For this review, take the finished solid that the model builds, in its own axes (mm). Coordinates: 2 decimals unless noted, no trailing zeros. Loops run counter-clockwise (first coordinate to the right, second up) from the corner with the lowest first, then second, coordinate; pieces in that order, holes last. Notation, with made-up numbers: (11.5, -37) -> (16.5, -37) arc R27 ccw to (16.5, -16) -> close; hole circle Ø4 at (17, 4.25). An arc over 180 degrees is marked (long way). One line per item, written item: value.
from build123d import *

# Parameters (mm, degrees)
F0_W     = 238.19866
F0_H     = 266.7
F0_R     = 3.2639
F1_DEPTH = 4.7752
F2_SIZE  = 22.352


with BuildPart() as f1:
    # F0 (on Front) → F1 (new body)
    with BuildSketch(Plane.XZ):
        Rectangle(F0_W, F0_H)
        with Locations((-106.75493, -95.25)):
            Circle(F0_R, mode=Mode.SUBTRACT)
        with Locations((-106.75493, -44.45)):
            Circle(F0_R, mode=Mode.SUBTRACT)
        with Locations((106.75493, -95.25)):
            Circle(F0_R, mode=Mode.SUBTRACT)
        with Locations((106.75493, -44.45)):
            Circle(F0_R, mode=Mode.SUBTRACT)
        with Locations((-106.75493, 0)):
            Circle(F0_R, mode=Mode.SUBTRACT)
        with Locations((-106.75493, 44.45)):
            Circle(F0_R, mode=Mode.SUBTRACT)
        with Locations((-106.75493, 88.9)):
            Circle(F0_R, mode=Mode.SUBTRACT)
        with Locations((106.75493, 0)):
            Circle(F0_R, mode=Mode.SUBTRACT)
        with Locations((106.75493, 44.45)):
            Circle(F0_R, mode=Mode.SUBTRACT)
        with Locations((106.75493, 88.9)):
            Circle(F0_R, mode=Mode.SUBTRACT)
    extrude(amount=-F1_DEPTH)

    # F2
    f2_edges = [f1.edges().sort_by_distance(p)[0] for p in [
        (119.09933, 2.3876, 133.35),
        (-119.09933, 2.3876, 133.35),
    ]]
    chamfer(f2_edges, length=F2_SIZE)


solid = f1.part
1. Insertion check: pin 1 Ø5 at (x, z) = (106.75, 44.45) entering from +Y. The pin has a flat end and moves straight along its axis. Give the tip position at first contact, or say it passes through.
Return value:
pin 1: passes through
2. The part is to be moulded in two halves that separate along X. For faces 1 (the flat face through (-2, 0, 2)), 2 (the flat face through (-107.8, 2.4, 122.3)), 3 (the cylindrical face through (103.494, 2.354, 0.144)), say which applies: pulls with the +X half, pulls with the -X half, needs draft (parallel to the pull), parting line crosses it, or undercut.
Return value:
face 1: needs draft
face 2: pulls with the -X half
face 3: undercut
3. Take a section at A-A, the plane z = 44.45. Give the boundary of the cut face in (x, y).
Return value:
outline: (-119.1, 0) -> (-110.02, 0) -> (-110.02, 4.78) -> (-119.1, 4.78) -> close; (-103.49, 0) -> (103.49, 0) -> (103.49, 4.78) -> (-103.49, 4.78) -> close; (110.02, 0) -> (119.1, 0) -> (119.1, 4.78) -> (110.02, 4.78) -> close
4. To check wall thickness, follow probe 1 along Z at (x, y) = (-99.5, 3.95); probe 2 along Z at (x, y) = (102, 1.45). State the ranges of each line that lie inside material, in increasing order. Write a range as from..to.
Return value:
probe 1: z = -133.35..130.6
probe 2: z = -133.35..128.1
